Verification items for the finished model (mm, model axes). A direction names the side the tool comes from. Give positions to 0.01 mm unless a question says otherwise; leave off trailing zeros. Write each loop counter-clockwise with the first axis right and the second up, starting at its lowest first coordinate (ties: lowest second). Pieces come first, ordered by that corner, then holes. Notation, with made-up numbers: (18, 13) - (64, 13) arc R33 ccw to (64, 51) - close; hole circle Ø5 at (1, -29). An arc over 180 degrees is marked (long way). Answer as a JSON object with one key per item and string values. Group by question number.
Item 1: Scan lines: line 1 along X through (y, z) = (1.75, -39.25); line 2 along X through (y, z) = (3.75, -31); line 3 along Y through (x, z) = (-18, -45.5). Record each from-to range of solid material in increasing order. Write a range as [from, to].
Item 2: Sectioned sample at A-A, the plane x = -25. Record the boundary of the cut face in (y, z), and give its area (3 significant figures).
Item 3: Tool access check on faces 1 (the face through (-6.766, 5.07, -45.668)), 2 (the face through (36.43, 4.94, -32.95)), 3 (the face through (25.094, 5.07, -44.307)). Record the directions out of +Z, -Z, +X, -X, +Y, -Y that give a thin tool (end or side, any length) a straight path to the whole face; none if there is none.
Item 4: Go/stop test with flat-tipped pins: pin 1 (5 mm diameter, centred on y = 7.5, z = -44, fed in from +X); pin 2 (3 mm diameter, centred on x = -19.5, y = 5.5, fed in from -Z); pin 3 (3.5 mm diameter, centred on x = -0.5, y = 6.5, fed in from +Z). Record where each tip stops, or that it passes through.
Item 5: Draft check along Y on faces 4 (the face through (-37.28, 5.07, -30.21)), 5 (the face through (35.727, 4.944, -32.241)). Enter one of: +Y half, -Y half, draft (parallel to the pull), parting line (faces both ways), or undercut.
Item 6: Sectioned sample at B-B, the plane y = 5. Count the separate pieces of the cut face and the enclosed holes in it, and give its area (3 significant figures).
```python
from build123d import *

# Parameters (mm, degrees)
BOSS_EXTRUDE1_DEPTH = 10
CUT_EXTRUDE1_DEPTH  = 10
CIRPATTERN1_COUNT   = 13
CIRPATTERN1_ANGLE   = 84
CUT_EXTRUDE2_START  = -1
CUT_EXTRUDE2_DEPTH  = 8
SKETCH5_W           = 8
SKETCH5_H           = 10
SKETCH5_W_2         = 0.983564582
SKETCH5_H_2         = 7.885827621
BOSS_EXTRUDE2_DEPTH = 5
SKETCH6_W           = 8
SKETCH6_H           = 10
SKETCH6_W_2         = 1
SKETCH6_H_2         = 8
BOSS_EXTRUDE3_DEPTH = 5
SKETCH7_R           = 1.15
CUT_EXTRUDE3_DEPTH  = 20
SKETCH9_R           = 1.15
CUT_EXTRUDE4_DEPTH  = 26
SKETCH10_R          = 1.15
CUT_EXTRUDE5_DEPTH  = 26
BOSS_EXTRUDE4_DEPTH = 10
CUT_EXTRUDE7_DEPTH  = 26


with BuildPart() as part:
    # Sketch1 → Boss-Extrude1 (new body)
    with BuildSketch(Plane(origin=(0, 0, 0), x_dir=(1, 0, 0), z_dir=(0, 1, 0))):
        with BuildLine():
            Line((-31.50867817, 31.50867817), (-37.165532419, 37.165532419))
            ThreePointArc((-37.165532419, 37.165532419), (0, 52.56), (37.165532419, 37.165532419))
            Line((37.165532419, 37.165532419), (31.50867817, 31.50867817))
            ThreePointArc((31.50867817, 31.50867817), (0, 44.56), (-31.50867817, 31.50867817))
        make_face()
    extrude(amount=BOSS_EXTRUDE1_DEPTH)

    # Sketch3 → Cut-Extrude1 (cut)
    with BuildSketch(Plane(origin=(0, 10, 0), x_dir=(1, 0, 0), z_dir=(0, 1, 0))):
        with BuildLine():
            Line((-31.95767776, 35.492596865), (-31.50867817, 31.50867817))
            ThreePointArc((-31.50867817, 31.50867817), (-29.816459819, 33.114533423), (-28.042516625, 34.629624043))
            Line((-28.042516625, 34.629624043), (-31.95767776, 35.492596865))
        make_face()
        with BuildLine():
            Line((-33.02828673, 36.681628586), (-33.077079754, 40.846791734))
            ThreePointArc((-33.077079754, 40.846791734), (-35.16950467, 39.059692027), (-37.165532419, 37.165532419))
            Line((-37.165532419, 37.165532419), (-33.02828673, 36.681628586))
        make_face()
    cut_extrude1 = extrude(amount=-CUT_EXTRUDE1_DEPTH, mode=Mode.SUBTRACT)

    # CirPattern1: Cut-Extrude1 ×13 about axis
    cirpattern1_axis = Axis((0, 0, 0), (0, -1, 0))
    for i in range(1, CIRPATTERN1_COUNT):
        add(cut_extrude1.rotate(cirpattern1_axis, i * CIRPATTERN1_ANGLE / (CIRPATTERN1_COUNT - 1)), mode=Mode.SUBTRACT)

    # Sketch4 → Cut-Extrude2 (cut)
    with BuildSketch(Plane(origin=(0, 10, 0), x_dir=(1, 0, 0), z_dir=(0, 1, 0)).offset(CUT_EXTRUDE2_START)):
        with BuildLine():
            Line((33.983551904, 33.983551904), (34.690658685, 34.690658685))
            ThreePointArc((34.690658685, 34.690658685), (0, 49.06), (-34.690658685, 34.690658685))
            Line((-34.690658685, 34.690658685), (-33.983551904, 33.983551904))
            ThreePointArc((-33.983551904, 33.983551904), (0, 48.06), (33.983551904, 33.983551904))
        make_face()
    extrude(amount=-CUT_EXTRUDE2_DEPTH, mode=Mode.SUBTRACT)

    # Sketch5 → Boss-Extrude2 (add)
    with BuildSketch(Plane(origin=(0, 0, 0), x_dir=(0.707106781, 0, 0.707106781), z_dir=(-0.707106781, 0, 0.707106781))):
        with Locations((-48.56, 5)):
            Rectangle(SKETCH5_W, SKETCH5_H)
        with Locations((-48.568217709, 5.057086189)):
            Rectangle(SKETCH5_W_2, SKETCH5_H_2, mode=Mode.SUBTRACT)
    extrude(amount=BOSS_EXTRUDE2_DEPTH)

    # Sketch6 → Boss-Extrude3 (add)
    with BuildSketch(Plane(origin=(0, 0, 0), x_dir=(0.707106781, 0, -0.707106781), z_dir=(0.707106781, 0, 0.707106781))):
        with Locations((48.56, 5)):
            Rectangle(SKETCH6_W, SKETCH6_H)
        with Locations((48.56, 5)):
            Rectangle(SKETCH6_W_2, SKETCH6_H_2, mode=Mode.SUBTRACT)
    extrude(amount=BOSS_EXTRUDE3_DEPTH)

    # Sketch7 → Cut-Extrude3 (cut)
    with BuildSketch(Plane(origin=(0, 10, 0), x_dir=(1, 0, 0), z_dir=(0, 1, 0))):
        with Locations((-3.086614159, 50.465695408)):
            Circle(SKETCH7_R)
        with Locations((3.086614159, 50.465695408)):
            Circle(SKETCH7_R)
    extrude(amount=-CUT_EXTRUDE3_DEPTH, mode=Mode.SUBTRACT)

    # Sketch9 → Cut-Extrude4 (cut)
    with BuildSketch(Plane(origin=(0, 10, 0), x_dir=(1, 0, 0), z_dir=(0, 1, 0))):
        with Locations((34.832080041, 30.589439354)):
            Circle(SKETCH9_R)
    extrude(amount=-CUT_EXTRUDE4_DEPTH, mode=Mode.SUBTRACT)

    # Sketch10 → Cut-Extrude5 (cut)
    with BuildSketch(Plane(origin=(0, 10, 0), x_dir=(1, 0, 0), z_dir=(0, 1, 0))):
        with Locations((-34.832080041, 30.589439354)):
            Circle(SKETCH10_R)
    extrude(amount=-CUT_EXTRUDE5_DEPTH, mode=Mode.SUBTRACT)

    # Sketch11 → Boss-Extrude4 (add)
    with BuildSketch(Plane(origin=(0, 10, 0), x_dir=(1, 0, 0), z_dir=(0, 1, 0))):
        Polygon((-2.75077786, 52.487968347), (2.75077786, 52.487968347), (0, 49.36), align=None)
        Polygon((0, 47.76), (-2.33209021, 44.498932069), (2.33209021, 44.498932069), align=None)
    extrude(amount=-BOSS_EXTRUDE4_DEPTH)

    # Sketch14 → Cut-Extrude7 (cut)
    with BuildSketch(Plane(origin=(0, 10, 0), x_dir=(1, 0, 0), z_dir=(0, 1, 0))):
        Polygon((37.165532419, 37.165532419), (34.594853292, 34.594853292), (30.896603346, 38.293103238), (33.467282473, 40.863782365), align=None)
    extrude(amount=-CUT_EXTRUDE7_DEPTH, mode=Mode.SUBTRACT)


solid = part.part
```
Geometry check:
{
 "1": {"line 1": "[-33.06, -29.43], [-27.73, -22.81], [22.81, 27.73], [29.43, 31.85]", "line 2": "[-36.99, -35.91], [-33.76, -32.02], [32.02, 33.76], [35.91, 36.97]", "line 3": "[0, 1], [9, 10]"},
 "2": {"outline": "(0, -44.27) - (10, -44.27) - (10, -38.28) - (0, -38.28) - close; hole (1, -42.21) - (9, -42.21) - (9, -41.05) - (1, -41.05) - close", "area": "50.6 mm^2"},
 "3": {"face 1": "+Z, +Y, -Y", "face 2": "none", "face 3": "-Z, +Y, -Y"},
 "4": {"pin 1": "x = 28.19", "pin 2": "z = -47.82", "pin 3": "z = -44.5"},
 "5": {"face 4": "draft", "face 5": "undercut"},
 "6": {"separate pieces": "3", "enclosed holes": "4", "area": "383 mm^2"}
}
